Geometry check sheet. Reference: the model listing, model coordinates, mm. Give positions to 0.01 mm unless a question says otherwise; leave off trailing zeros. Order: outer loops, then holes, each group sorted by start corner. A loop starts at its lowest first (then second) coordinate and runs counter-clockwise, first axis right, second up. Notation, with made-up numbers: M 63,47 L 102,47 A27 cw 102,70 Z; hole C 64.5,65.5 d2. An arc over 180 degrees is marked long. Answer as CSV lines item,"result". Start each with the question number.
Q1. Section check C-C, the plane z = 1.5. Record the boundary of the cut face in (x, y), then the cut area to 3 significant figures.
Q2. Section check B-B, the plane x = 4.5. Record the boundary of the cut face in (y, z), then the cut area to 3 significant figures.
Q3. Thickness scan on line 1 (X direction, y = 457, z = -1.5); line 2 (Z direction, x = -8, y = 496.5). Record the ranges inside material, lowest first.
Q4. Section check A-A, the plane y = 538.5. Record the boundary of the cut face in (x, z).
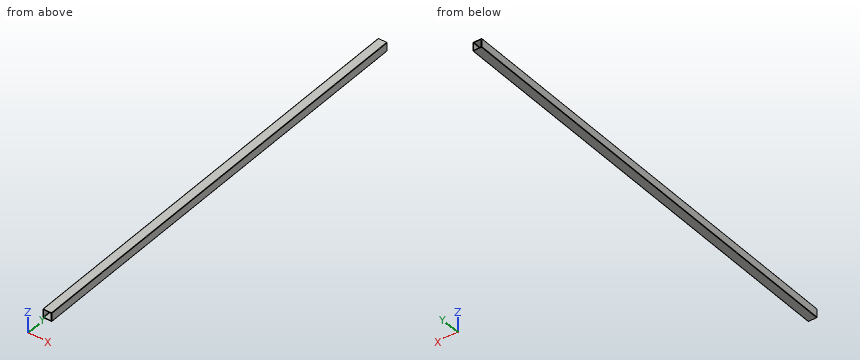
```python
from build123d import *

# Parameters (mm, degrees)
BOSS_EXTRUDE1_DEPTH = 1200
SKETCH2_W           = 101.895059676
SKETCH2_H           = 138.127514373
CUT_EXTRUDE1_DEPTH  = 220


with BuildPart() as part:
    # Sketch1 → Boss-Extrude1 (new body)
    with BuildSketch(Plane(origin=(0, 0, 0), x_dir=(1, 0, 0), z_dir=(0, 1, 0))):
        with BuildLine():
            Line((-9, -10), (9, -10))
            ThreePointArc((9, -10), (9.707106781, -9.707106781), (10, -9))
            Line((10, -9), (10, 9))
            ThreePointArc((10, 9), (9.707106781, 9.707106781), (9, 10))
            Line((9, 10), (-9, 10))
            ThreePointArc((-9, 10), (-9.707106781, 9.707106781), (-10, 9))
            Line((-10, 9), (-10, -9))
            ThreePointArc((-10, -9), (-9.707106781, -9.707106781), (-9, -10))
        make_face()
        with BuildLine():
            Line((-7.5, -8.5), (7.5, -8.5))
            ThreePointArc((7.5, -8.5), (8.207106781, -8.207106781), (8.5, -7.5))
            Line((8.5, -7.5), (8.5, 7.5))
            ThreePointArc((8.5, 7.5), (8.207106781, 8.207106781), (7.5, 8.5))
            Line((7.5, 8.5), (-7.5, 8.5))
            ThreePointArc((-7.5, 8.5), (-8.207106781, 8.207106781), (-8.5, 7.5))
            Line((-8.5, 7.5), (-8.5, -7.5))
            ThreePointArc((-8.5, -7.5), (-8.207106781, -8.207106781), (-7.5, -8.5))
        make_face(mode=Mode.SUBTRACT)
    extrude(amount=BOSS_EXTRUDE1_DEPTH)

    # Sketch2 → Cut-Extrude1 (cut)
    with BuildSketch(Plane.XZ):
        with Locations((4.315799724, -16.6218454)):
            Rectangle(SKETCH2_W, SKETCH2_H)
    extrude(amount=-CUT_EXTRUDE1_DEPTH, mode=Mode.SUBTRACT)


solid = part.part
```
Answer block:
1,outline,"M -10,220 L -8.5,220 L -8.5,1200 L -10,1200 Z; M 8.5,220 L 10,220 L 10,1200 L 8.5,1200 Z"
1,area,"2,940 mm2"
2,outline,"M 220,-10 L 1200,-10 L 1200,-8.5 L 220,-8.5 Z; M 220,8.5 L 1200,8.5 L 1200,10 L 220,10 Z"
2,area,"2,940 mm2"
3,line 1,"x = -10 to -8.5, 8.5 to 10"
3,line 2,"z = -10 to -8.37, 8.37 to 10"
4,outline,"M -10,-9 A1 ccw -9,-10 L 9,-10 A1 ccw 10,-9 L 10,9 A1 ccw 9,10 L -9,10 A1 ccw -10,9 Z; hole M -8.5,-7.5 A1 ccw -7.5,-8.5 L 7.5,-8.5 A1 ccw 8.5,-7.5 L 8.5,7.5 A1 ccw 7.5,8.5 L -7.5,8.5 A1 ccw -8.5,7.5 Z"
